The model under review builds one solid part; all positions refer to its coordinate system, in mm. A direction names the side the tool comes from. Give positions to 0.01 mm unless a question says otherwise; leave off trailing zeros. Order: outer loops, then holes, each group sorted by start corner. A loop starts at its lowest first (then second) coordinate and runs counter-clockwise, first axis right, second up. Notation, with made-up numbers: (36.25, 28.5) - (76.25, 28.5) arc R21 ccw to (76.25, 33.5) - close; hole circle Ø11 at (34.25, 87). An arc over 180 degrees is marked (long way). Use CSV: the item, a comma, the result in double quotes. Start each with the question number.
1. Machinability: for faces 4 (the flat face through (-21, 4.788, 13)), 5 (the flat face through (22, 4.788, 13)), 6 (the flat face through (-31.555, 2, 13)), which of the approach directions +Z, -Z, +X, -X, +Y, -Y give a long, thin tool a straight path to every point of the face, cutting with its end or side? Answer none if there is none.
2. Take a section at D-D, the plane z = 12.5. State the section outline as (x, y) points, then the cut area to 3 significant figures.
3. Take a section at A-A, the plane z = 7.25. State the section outline as (x, y) points.
4. To check wall thickness, follow line 1 (Y direction, x = -22, z = 14.5); line 2 (X direction, y = 3.5, z = 21.75); line 3 (X direction, y = 5.75, z = 9.5). State the ranges of each line that lie inside material, in increasing order. Write a range as [from, to].
5. For pin 1 (3 mm diameter, centred on x = -9, y = 6, fed in from -Z); pin 2 (6 mm diameter, centred on x = -16.32, z = 7.46, fed in from +Y); pin 3 (4 mm diameter, centred on y = 7, z = 4, fed in from +X); pin 4 (3.5 mm diameter, centred on x = 16.7, z = 7.46, fed in from +Y), all flat-tipped, find the tip position at first contact; note any pin that passes through.
6. Take a section at C-C, the plane y = 5.5. State the section outline as (x, z) points.
7. Take a section at B-B, the plane y = 2.5. State the section outline as (x, z) points (1 decimal), then the cut area to 3 significant figures.
8. Draft analysis for pull direction X (two halves, no side actions). For faces 1 (the flat face through (31.945, 2, 13)), 2 (the cylindrical face through (0.019, 7.706, 13.068)), 3 (the flat face through (0, 9, 26.507)), state which applies: released by +X, released by -X, zero draft, split by the parting line, or undercut.
```python
from build123d import *

# Parameters (mm, degrees)
BOSS_EXTRUDE2_DEPTH    = 26.50744
CUT_EXTRUDE1_START     = -0.02543021
CUT_EXTRUDE1_OUTLINE_W = 66
CUT_EXTRUDE1_OUTLINE_H = 16
CUT_EXTRUDE1_DEPTH     = 1.106877933
CUT_EXTRUDE2_REACH     = 45.41
SKETCH4_R              = 2.2225


# Read off the part's stored shape, not the designer's step: Cut-Extrude1
with BuildPart() as part:
    # Sketch2 → Boss-Extrude2 (new body)
    with BuildSketch(Plane.XY):
        with BuildLine():
            ThreePointArc((-11.445222977, 4.788221067), (-12.237590886, 2.302953542), (-12.505480711, -0.291778933))
            Line((-12.505480711, -0.291778933), (-7.805480711, -0.291778933))
            ThreePointArc((-7.805480711, -0.291778933), (0.194519289, 7.708221067), (8.194519289, -0.291778933))
            Line((8.194519289, -0.291778933), (12.894519289, -0.291778933))
            ThreePointArc((12.894519289, -0.291778933), (12.626629463, 2.302953542), (11.834261554, 4.788221067))
            ThreePointArc((11.834261554, 4.788221067), (0.194519289, 12.408221067), (-11.445222977, 4.788221067))
        make_face()
        with BuildLine():
            Line((-31.555480711, -0.291778933), (-12.505480711, -0.291778933))
            ThreePointArc((-12.505480711, -0.291778933), (-12.237590886, 2.302953542), (-11.445222977, 4.788221067))
            Line((-11.445222977, 4.788221067), (-31.555480711, 4.788221067))
            Line((-31.555480711, 4.788221067), (-31.555480711, -0.291778933))
        make_face()
        with BuildLine():
            ThreePointArc((11.834261554, 4.788221067), (12.626629463, 2.302953542), (12.894519289, -0.291778933))
            Line((12.894519289, -0.291778933), (31.944519289, -0.291778933))
            Line((31.944519289, -0.291778933), (31.944519289, 4.788221067))
            Line((31.944519289, 4.788221067), (11.834261554, 4.788221067))
        make_face()
    extrude(amount=BOSS_EXTRUDE2_DEPTH)

    # Cut-Extrude1 outline → Cut-Extrude1 (cut)
    with BuildSketch(Plane(origin=(0, 0, 0), x_dir=(1, 0, 0), z_dir=(0, 0.08715574274765836, -0.9961946980917455)).offset(CUT_EXTRUDE1_START)):
        with Locations((0, -6)):
            Rectangle(CUT_EXTRUDE1_OUTLINE_W, CUT_EXTRUDE1_OUTLINE_H)
    extrude(amount=CUT_EXTRUDE1_DEPTH, mode=Mode.SUBTRACT)

    # Sketch4 → Cut-Extrude2 (cut, up to next)
    with BuildSketch(Plane.XZ.offset(0.291778933), mode=Mode.PRIVATE) as cut_extrude2_sk1:
        with Locations(Location((-16.315480711, 7.45744, 0), (0, 0, 270))):
            Circle(SKETCH4_R)
    cut_extrude2_tool1 = extrude(cut_extrude2_sk1.sketch, amount=-CUT_EXTRUDE2_REACH, mode=Mode.PRIVATE) & part.part
    # Sketch4 → Cut-Extrude2 (cut, up to next)
    with BuildSketch(Plane.XZ.offset(0.291778933), mode=Mode.PRIVATE) as cut_extrude2_sk2:
        with Locations(Location((16.704519289, 7.45744, 0), (0, 0, 270))):
            Circle(SKETCH4_R)
    cut_extrude2_tool2 = extrude(cut_extrude2_sk2.sketch, amount=-CUT_EXTRUDE2_REACH, mode=Mode.PRIVATE) & part.part
    add(cut_extrude2_tool1.solids().sort_by_distance((-16.315481, -0.291779, 7.45744))[0], mode=Mode.SUBTRACT)
    add(cut_extrude2_tool2.solids().sort_by_distance((16.704519, -0.291779, 7.45744))[0], mode=Mode.SUBTRACT)


solid = part.part
```
Determined:
1,face 4,"+Z, -Z, -X, +Y"
1,face 5,"+Z, -Z, +X, +Y"
1,face 6,"+Z, -Z, -X, +Y, -Y"
2,outline,"(-31.56, -0.29) - (-7.81, -0.29) arc R8 cw to (8.19, -0.29) - (31.94, -0.29) - (31.94, 4.79) - (11.83, 4.79) arc R12.7 ccw to (-11.45, 4.79) - (-31.56, 4.79) - close"
2,area,"350 mm²"
3,outline,"(-31.56, -0.29) - (-18.53, -0.29) - (-18.53, 4.79) - (-31.56, 4.79) - close; (-14.1, -0.29) - (-7.81, -0.29) arc R8 cw to (8.19, -0.29) - (14.49, -0.29) - (14.49, 4.79) - (11.83, 4.79) arc R12.7 ccw to (-11.45, 4.79) - (-14.1, 4.79) - close; (18.92, -0.29) - (31.94, -0.29) - (31.94, 4.79) - (18.92, 4.79) - close"
4,line 1,"y = [-0.29, 4.79]"
4,line 2,"x = [-31.56, -6.85], [7.24, 31.94]"
4,line 3,"x = [-10.98, -5.05], [5.44, 11.37]"
5,pin 1,"stops at z = 0.42"
5,pin 2,"stops at y = 4.79"
5,pin 3,"stops at x = 11.74"
5,pin 4,"passes through"
6,outline,"(-11.11, 0.51) - (-5.32, 0.51) - (-5.32, 26.51) - (-11.11, 26.51) - close; (5.71, 0.51) - (11.5, 0.51) - (11.5, 26.51) - (5.71, 26.51) - close"
7,outline,"(-31.6, 0.2) - (-7.3, 0.2) - (-7.3, 26.5) - (-31.6, 26.5) - close; (7.7, 0.2) - (31.9, 0.2) - (31.9, 26.5) - (7.7, 26.5) - close; hole circle Ø4.4 at (-16.3, 7.5); hole circle Ø4.4 at (16.7, 7.5)"
7,area,"1,240 mm²"
8,face 1,"released by +X"
8,face 2,"undercut"
8,face 3,"zero draft"
